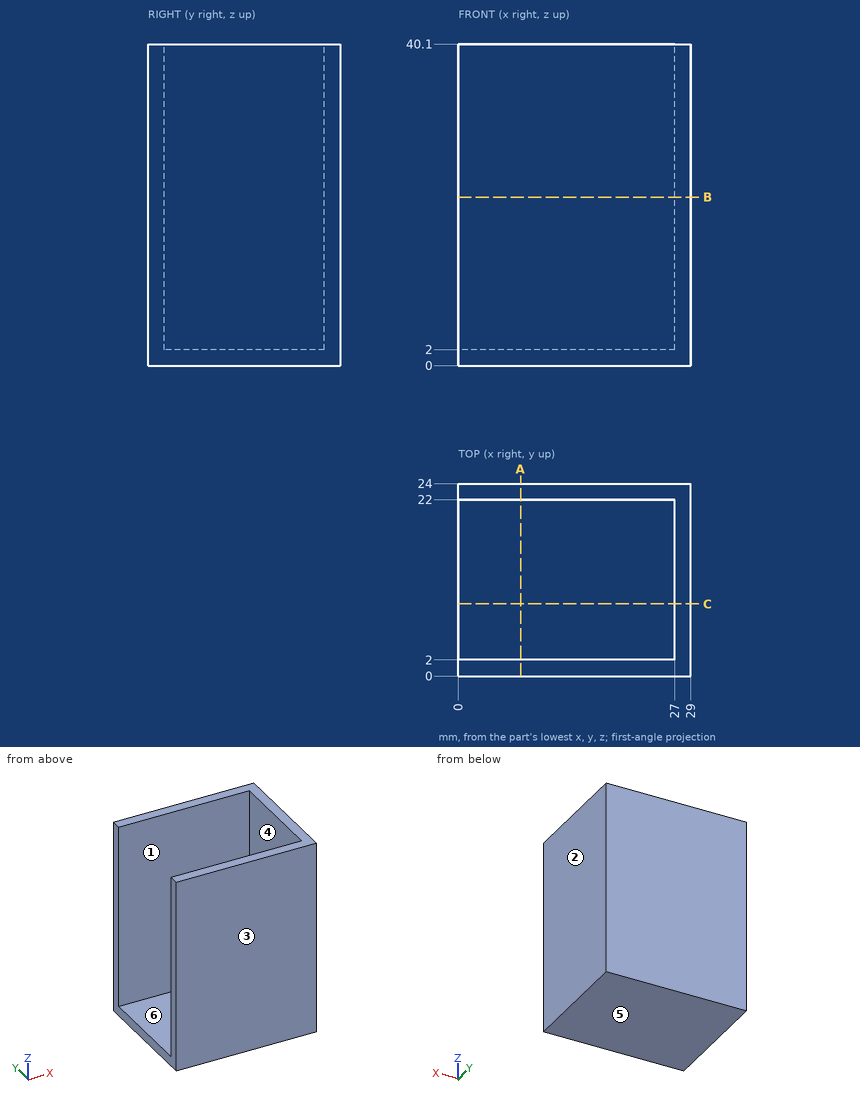
Here's the drawing with two shaded views (mm, measured from the low corner). I have some questions. A direction names the side the tool comes from. Give positions to 0.01 mm unless a question says otherwise; leave off trailing zeros. Loops run counter-clockwise (first coordinate to the right, second up) from the corner with the lowest first, then second, coordinate; pieces in that order, holes last. Notation, with made-up numbers: (-1.75, 44.5) - (15.25, 44.5) arc R30 ccw to (15.25, 73.5) - close; hole circle Ø7 at (3, 72). An arc over 180 degrees is marked (long way). Answer in a Markdown table with one row per item. Add a question column.
Q1. For pin 1 (6 mm diameter, centred on y = 17.5, z = 15, fed in from -X); pin 2 (8 mm diameter, centred on x = 13.5, z = 6.5, fed in from -Y); pin 3 (1.5 mm diameter, centred on x = 3.5, y = 16, fed in from +Z), each with a flat end and sliding along its axis, tell me the tip position at first contact or that it passes through.
Q2. We'd pull the mould along Y, two halves only. Please class the marked faces 1, 2, 3 and 4: +Y half, -Y half, draft (parallel to the pull), parting line (faces both ways), or undercut.
Q3. Please list where these lines run through material, in increasing order: L1, parallel to Y at x = 19, z = 10.5; L2, parallel to Z at x = 6.5, y = 3.25; L3, parallel to X at y = 13, z = 25.5. Write a range as from..to.
Q4. Which directions (+Z, -Z, +X, -X, +Y, -Y) give clear straight access to the entire face, cutting with the end or side of a thin tool? Please do the marked faces 5 and 6.
Q5. If we section it at C-C (y = 9): List the corners of the cut face in (x, z) for me.
Q6. If we section it at A-A (x = 7.75): List the corners of the cut face in (y, z) for me.
Q7. If we section it at B-B (z = 21): List the corners of the cut face in (x, y) for me.
The answers:
| question | item | result |
|---|---|---|
| 1 | pin 1 | stops at x = 27 |
| 1 | pin 2 | stops at y = 0 |
| 1 | pin 3 | stops at z = 2 |
| 2 | face 1 | undercut |
| 2 | face 2 | draft |
| 2 | face 3 | -Y half |
| 2 | face 4 | undercut |
| 3 | L1 | y = 0..2, 22..24 |
| 3 | L2 | z = 0..2 |
| 3 | L3 | x = 27..29 |
| 4 | face 5 | -Z, +X, -X, +Y, -Y |
| 4 | face 6 | +Z, -X |
| 5 | outline | (0, 0) - (29, 0) - (29, 40.1) - (27, 40.1) - (27, 2) - (0, 2) - close |
| 6 | outline | (0, 0) - (24, 0) - (24, 40.1) - (22, 40.1) - (22, 2) - (2, 2) - (2, 40.1) - (0, 40.1) - close |
| 7 | outline | (0, 0) - (29, 0) - (29, 24) - (0, 24) - (0, 22) - (27, 22) - (27, 2) - (0, 2) - close |
